Geometry check sheet. Reference: drawing and pictorial views, mm from the part's lowest x, y, z. Round coordinates to 2 decimals unless told otherwise and drop trailing zeros. Order: outer loops, then holes, each group sorted by start corner. A loop starts at its lowest first (then second) coordinate and runs counter-clockwise, first axis right, second up.
(1) Sectioned sample at A-A (x = 25). Record the boundary of the cut face in (y, z).
(2) Sectioned sample at C-C (y = 36). Record the boundary of the cut face in (x, z).
(3) Sectioned sample at D-D (z = 43.5). Record the boundary of the cut face in (x, y).
(4) Release check for a two-part mould opening along X. For the marked faces 1, 2 and 3 record: +X half, -X half, draft (parallel to the pull), parting line (faces both ways), or undercut.
(5) Material ranges on line 1 along Z through (x, y) = (42, 22.5); line 2 along X through (y, z) = (12, 15.5) (1 decimal); line 3 along Y through (x, z) = (25, 21.5), recorded low to high.
(6) Go/stop test with flat-tipped pins: pin 1 (13.5 mm diameter, centred on x = 24, y = 33.5, fed in from +Z); pin 2 (6 mm diameter, centred on x = 25, y = 25, fed in from +Z); pin 3 (12 mm diameter, centred on x = 42, z = 37, fed in from +Y); pin 4 (1 mm diameter, centred on x = 32.5, z = 24.5, fed in from +Y). Record where each tip stops, or that it passes through.
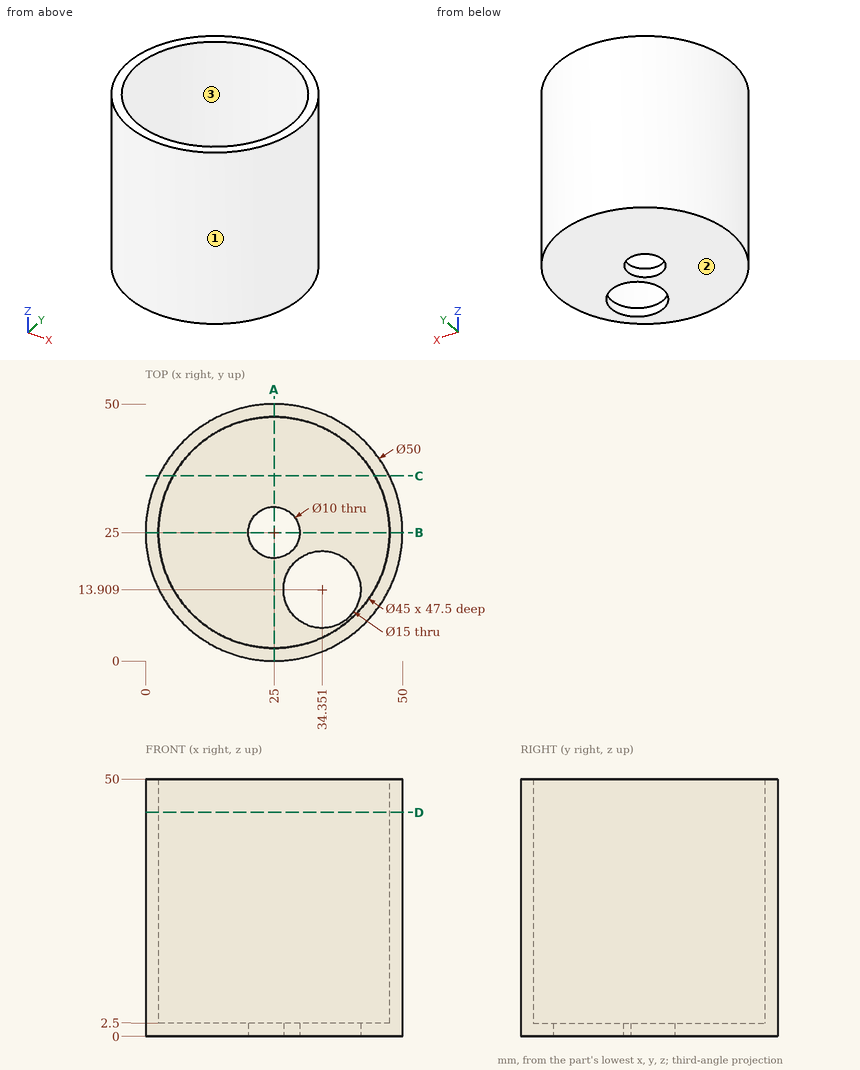
Answer below:
1. outline: (0, 0) - (20, 0) - (20, 2.5) - (2.5, 2.5) - (2.5, 50) - (0, 50) - close; (30, 0) - (50, 0) - (50, 50) - (47.5, 50) - (47.5, 2.5) - (30, 2.5) - close
2. outline: (2.55, 0) - (47.45, 0) - (47.45, 50) - (44.63, 50) - (44.63, 2.5) - (5.37, 2.5) - (5.37, 50) - (2.55, 50) - close
3. outline: circle Ø50 at (25, 25); hole circle Ø45 at (25, 25)
4. face 1: parting line
4. face 2: draft
4. face 3: undercut
5. line 1: z = 0 to 2.5
5. line 2: x = 3.6 to 6.6, 43.4 to 46.4
5. line 3: y = 0 to 2.5, 47.5 to 50
6. pin 1: stops at z = 2.5
6. pin 2: passes through
6. pin 3: stops at y = 47.45
6. pin 4: stops at y = 49
